Model file for the job. Use its own axes, mm. Face numbers are marked on the shaded views. A direction names the side the tool comes from. Round coordinates to 2 decimals unless told otherwise and drop trailing zeros. Loops run counter-clockwise (first coordinate to the right, second up) from the corner with the lowest first, then second, coordinate; pieces in that order, holes last. Notation, with made-up numbers: (25.25, -2.5) -> (46.25, -2.5) arc R12 ccw to (46.25, 10.5) -> close; hole circle Ø7 at (-38.5, 16). An arc over 180 degrees is marked (long way). Use a Markdown table: item, result.
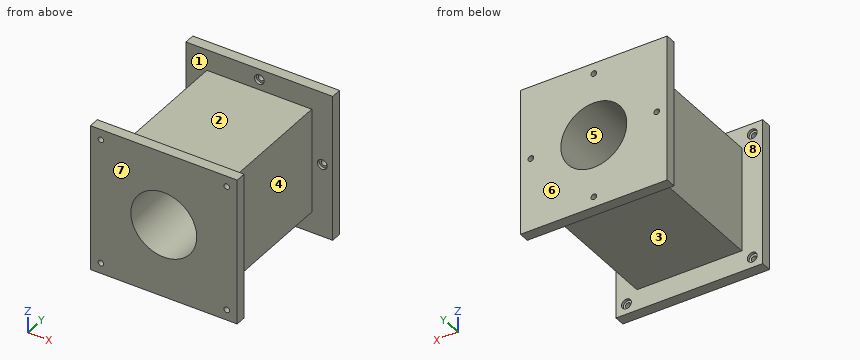
from build123d import *

# Parameters (mm, degrees)
SKETCH1_W           = 177.8
SKETCH1_H           = 177.8
BOSS_EXTRUDE1_DEPTH = 12.7
LPATTERN1_COUNT     = 2
LPATTERN1_PITCH     = 177.8
CIRPATTERN1_COUNT   = 4
CIRPATTERN2_COUNT   = 4
BOSS_EXTRUDE2_REACH = 219.76
SKETCH11_W          = 127
SKETCH11_H          = 127
SKETCH12_R          = 39.925273759
CUT_EXTRUDE1_DEPTH  = 229.246949596


with BuildPart() as part:
    # Sketch1 → Boss-Extrude1 (new body)
    with BuildSketch(Plane(origin=(0, 0, 0), x_dir=(1, 0, 0), z_dir=(0, 1, 0))):
        Rectangle(SKETCH1_W, SKETCH1_H)
    extrude(amount=BOSS_EXTRUDE1_DEPTH)


with BuildPart() as lpattern1_1:
    # LPattern1: pattern copy
    add(part.part.moved(Location(Vector(0, 1, 0) * (1 * LPATTERN1_PITCH))))

    # Sketch10 → CBORE for 1_4 Button Head Cap Screw2 (revolve, cut)
    with BuildSketch(Plane(origin=(76.2, 177.8, 0), x_dir=(0, 0, -1), z_dir=(1, 0, 0))):
        Polygon((0, 0), (0, 12.7), (3.3782, 12.7), (3.3782, 3.3528), (5.95376, 3.3528), (5.95376, 0), align=None)
    cbore_for_1_4_button_head_cap_screw2 = revolve(axis=Axis((76.2, 171.45, 0), (0, 1, 0)), mode=Mode.SUBTRACT)

    # CirPattern2: CBORE for 1_4 Button Head Cap Screw2 ×4 about axis
    cirpattern2_axis = Axis((0, 0, 0), (0, 1, 0))
    for i in range(1, CIRPATTERN2_COUNT):
        add(cbore_for_1_4_button_head_cap_screw2.rotate(cirpattern2_axis, i * 360 / CIRPATTERN2_COUNT), mode=Mode.SUBTRACT)

    # Sketch11 → Boss-Extrude2 (add, up to next)
    with BuildSketch(Plane(origin=(0, 12.7, 0), x_dir=(1, 0, 0), z_dir=(0, 1, 0)), mode=Mode.PRIVATE) as boss_extrude2_sk1:
        Rectangle(SKETCH11_W, SKETCH11_H)
    boss_extrude2_tool1 = extrude(boss_extrude2_sk1.sketch, amount=BOSS_EXTRUDE2_REACH, mode=Mode.PRIVATE) - lpattern1_1.part


with BuildPart() as part_1:
    add(part.part)

    # Sketch5 → CBORE for 1_4 Button Head Cap Screw1 (revolve, cut)
    with BuildSketch(Plane(origin=(76.2, 12.7, -76.2), x_dir=(0, 0, 1), z_dir=(1, 0, 0))):
        Polygon((0, 0), (0, 12.7), (3.3782, 12.7), (3.3782, 3.3528), (5.95376, 3.3528), (5.95376, 0), align=None)
    cbore_for_1_4_button_head_cap_screw1 = revolve(axis=Axis((76.2, 19.05, -76.2), (0, -1, 0)), mode=Mode.SUBTRACT)

    # CirPattern1: CBORE for 1_4 Button Head Cap Screw1 ×4 about axis
    cirpattern1_axis = Axis((0, 0, 0), (0, 1, 0))
    for i in range(1, CIRPATTERN1_COUNT):
        add(cbore_for_1_4_button_head_cap_screw1.rotate(cirpattern1_axis, i * 360 / CIRPATTERN1_COUNT), mode=Mode.SUBTRACT)


with BuildPart() as lpattern1_1_1:
    add(lpattern1_1.part)

    add(part_1.part)  # Boss-Extrude2 merges part
    add(boss_extrude2_tool1.solids().sort_by_distance((0, 12.7, 0))[0])

    # Sketch12 → Cut-Extrude1 (cut, through all)
    with BuildSketch(Plane(origin=(0, 190.5, 0), x_dir=(1, 0, 0), z_dir=(0, 1, 0))):
        with Locations(Location((0, 0, 0), (0, 0, 270))):
            Circle(SKETCH12_R)
    extrude(amount=-CUT_EXTRUDE1_DEPTH, mode=Mode.SUBTRACT)


solid = lpattern1_1_1.part
Q1. Band-saw the part on C-C, the plane x = 51.5. Give the cut face in (y, z).
Results list:
| item | result |
|---|---|
| outline | (0, -88.9) -> (12.7, -88.9) -> (12.7, -63.5) -> (177.8, -63.5) -> (177.8, -88.9) -> (190.5, -88.9) -> (190.5, 88.9) -> (177.8, 88.9) -> (177.8, 63.5) -> (12.7, 63.5) -> (12.7, 88.9) -> (0, 88.9) -> close |
Q2. Band-saw the part on A-A, the plane x = -76.2. Give the number of separate pieces and of enclosed holes in the cut face, plus the area to 3 significant figures.
Results list:
| item | result |
|---|---|
| separate pieces | 5 |
| enclosed holes | 0 |
| area | 4,210 mm² |
Q3. Flat gauge pins, fed straight in: pin 1 (5.5 mm diameter, centred on x = -76.2, z = -76.2, fed in from -Y); pin 2 (12 mm diameter, centred on x = 14.5, y = 80.5, fed in from -Z); pin 3 (6 mm diameter, centred on x = 65, y = 149, fed in from +Z). Where does each tip first touch, or does it go through?
Results list:
| item | result |
|---|---|
| pin 1 | stops at y = 177.8 |
| pin 2 | stops at z = -63.5 |
| pin 3 | stops at z = 63.5 |
Q4. Pull direction Y, two halves, no side cores. Call the marked faces 5, 6, 7 and 8: released by +Y, released by -Y, zero draft, split by the parting line, or undercut.
Results list:
| item | result |
|---|---|
| face 5 | zero draft |
| face 6 | released by +Y |
| face 7 | released by -Y |
| face 8 | undercut |
Q5. Tool access for the marked faces 1, 2, 3 and 4: list every direction of +Z, -Z, +X, -X, +Y, -Y with a clear straight run to the whole face (end or side of a thin tool).
Results list:
| item | result |
|---|---|
| face 1 | none |
| face 2 | +Z, +X, -X |
| face 3 | -Z, +X, -X |
| face 4 | +Z, -Z, +X |
Q6. Drill centre lines: L1, parallel to X at y = 183.25, z = 0; L2, parallel to Z at x = 76, y = 3; L3, parallel to X at y = 90, z = 0. Where is each one in solid material? Low to high. Write a range as from..to.
Results list:
| item | result |
|---|---|
| L1 | x = -88.9..-79.58, -72.82..-39.93, 39.93..72.82, 79.58..88.9 |
| L2 | z = -88.9..-79.57, -72.83..72.83, 79.57..88.9 |
| L3 | x = -63.5..-39.93, 39.93..63.5 |
